Model file for the job. Use its own axes, mm. A direction names the side the tool comes from. Round coordinates to 2 decimals unless told otherwise and drop trailing zeros. Order: outer loops, then holes, each group sorted by start corner. A loop starts at its lowest first (then second) coordinate and runs counter-clockwise, first axis right, second up. Notation, with made-up numbers: (14, 87.5) -> (19, 87.5) arc R23 ccw to (19, 111.5) -> close; hole circle Ø1 at (85, 36). An arc over 180 degrees is marked (long way). Answer as CSV lines item,"result".
```python
from build123d import *

# Parameters (mm, degrees)
RADYUS2_R = 2
PAH1_SIZE = 1
IZIM2_W   = 0.487804803
IZIM2_H   = 8


with BuildPart() as part:
    # Çizim1 → Döndür1 (revolve)
    with BuildSketch(Plane.XY, mode=Mode.PRIVATE) as d_nd_r1_sk:
        Polygon((0, 0), (0, 7), (43, 7), (43, 17.5), (48, 17.5), (48, 12.5), (53, 12.5), (53, 7), (58, 7), (58, 8), (72, 8), (72, 0), align=None)
    revolve(d_nd_r1_sk.sketch.rotate(Axis((0, 0, 0), (1, 0, 0)), 90), axis=Axis((0, 0, 0), (1, 0, 0)))

    # Radyus2
    # the kernel refuses this fillet: 2 mm, written as the material it adds along each edge
    with BuildSketch(Plane(origin=(58, 0, 0), x_dir=(0, 0, 1), z_dir=(0, 1, 0))) as radyus2_piece_1:
        with BuildLine():
            CenterArc((9, -1.732050808), RADYUS2_R, 120, 60)
            Line((8, 0), (7.98, 0.034641016))
            ThreePointArc((7.98, 0.034641016), (7.5, 0.04), (7, 0.04))
            Line((7, 0.04), (6.96, 0))
            Line((6.96, 0), (6.96, -1.732050808))
            Line((6.96, -1.732050808), (7, -1.732050808))
        make_face()
    revolve(axis=Axis((58, 0, 0), (1, 0, 0)))
    with BuildSketch(Plane(origin=(53, 0, 0), x_dir=(0, 0, 1), z_dir=(0, 1, 0))) as radyus2_piece_2:
        with BuildLine():
            CenterArc((7 + RADYUS2_R, RADYUS2_R), RADYUS2_R, 180, 90)
            Line((7, RADYUS2_R), (7 - RADYUS2_R * 0.02, RADYUS2_R))
            Line((7 - RADYUS2_R * 0.02, RADYUS2_R), (7 - RADYUS2_R * 0.02, -RADYUS2_R * 0.02))
            Line((7 - RADYUS2_R * 0.02, -RADYUS2_R * 0.02), (7 + RADYUS2_R, -RADYUS2_R * 0.02))
            Line((7 + RADYUS2_R, -RADYUS2_R * 0.02), (7 + RADYUS2_R, 0))
        make_face()
    revolve(axis=Axis((53, 0, 0), (1, 0, 0)))

    # Pah1
    pah1_edges = [part.edges().sort_by_distance(p)[0] for p in [
        (0, 0, -7),
    ]]
    chamfer(pah1_edges, length=PAH1_SIZE)

    # Çizim2 → Kes-Döndür1 (revolve, cut)
    with BuildSketch(Plane.XY):
        with BuildLine():
            Line((69.5, 8), (72, 8))
            Line((72, 8), (72, 0))
            ThreePointArc((72, 0), (71.360443691, 4.190763654), (69.5, 8))
        make_face()
        with Locations((72.243902402, 4)):
            Rectangle(IZIM2_W, IZIM2_H)
    revolve(axis=Axis((72, 0, 0), (-1, 0, 0)), mode=Mode.SUBTRACT)


solid = part.part
```
Q1. Mould opens along X. For faces 4 (the flat face through (0, 0, 0)), 5 (the cylindrical face through (50.535, -3.755, 11.923)), 6 (the flat face through (48, 8, 11)), 7 (the cylindrical face through (55.64, 6.21, 3.23)) say: +X half, -X half, draft (parallel to the pull), parting line (faces both ways), or undercut.
Checks:
face 4,"-X half"
face 5,"draft"
face 6,"+X half"
face 7,"undercut"
Q2. Flat gauge pins, fed straight in: pin 1 (6 mm diameter, centred on y = 14, z = -10, fed in from -X); pin 2 (5 mm diameter, centred on x = 60.5, y = 11.5, fed in from +Z); pin 3 (10 mm diameter, centred on x = 43.5, z = -8.5, fed in from -Y); pin 4 (6 mm diameter, centred on x = 14, z = 8, fed in from -Y). Where does each tip first touch, or does it go through?
Checks:
pin 1,"x = 43"
pin 2,"through"
pin 3,"y = -17.15"
pin 4,"y = -4.9"
Q3. Wall check: L1, parallel to X at y = 9, z = -6.5; L2, parallel to X at y = -13, z = -9; L3, parallel to Y at x = 14.5, z = -0.5. Give the ranges that are in metal, low to high. Write a range as [from, to].
Checks:
L1,"[43, 53]"
L2,"[43, 48]"
L3,"[-6.98, 6.98]"
Q4. Saw through at D-D (z = 14). Write the cut outline in (x, y).
Checks:
outline,"(43, -10.5) -> (48, -10.5) -> (48, 10.5) -> (43, 10.5) -> close"
Q5. Saw through at A-A (z = 0). Write the cut outline in (x, y).
Checks:
outline,"(0, -6) -> (1, -7) -> (43, -7) -> (43, -17.5) -> (48, -17.5) -> (48, -12.5) -> (53, -12.5) -> (53, -9) arc R2 cw to (55, -7) -> (56.27, -7) arc R2 cw to (58, -8) -> (69.5, -8) arc R14.05 ccw to (69.5, 8) -> (58, 8) arc R2 cw to (56.27, 7) -> (55, 7) arc R2 cw to (53, 9) -> (53, 12.5) -> (48, 12.5) -> (48, 17.5) -> (43, 17.5) -> (43, 7) -> (1, 7) -> (0, 6) -> close"
Q6. Tool access for faces 1 (the flat face through (53, -3, -9)), 2 (the flat face through (43, 8, 0)), 3 (the cylindrical face through (45.535, 17.084, -3.794)): list every direction of +Z, -Z, +X, -X, +Y, -Y with a clear straight run to the whole face (end or side of a thin tool).
Checks:
face 1,"+X"
face 2,"-X"
face 3,"+X, -X"
Q7. Saw through at C-C (x = 16). Write the cut outline in (y, z).
Checks:
outline,"circle Ø14 at (0, 0)"
